The listing builds one solid part. Answer for the finished solid, in the listing's coordinates (mm). A direction names the side the tool comes from. Round coordinates to 2 decimals unless told otherwise and drop trailing zeros. Use a Markdown table: item, result. Add a question column.
Q1. Which of the six approach directions +Z, -Z, +X, -X, +Y, -Y give full straight-line access (tool end or side, diameter ignored) to faces 1 (the flat face through (104, 147, 2)), 2 (the flat face through (18.583, 98, 2)), 3 (the flat face through (231, 5, 2)), 4 (the flat face through (104, 2, 2))?
Q2. Section A-A on x = 191.5 is taken. Give the number of separate pieces and of enclosed holes in the cut face, then the cut area to 3 significant figures.
Q3. For a pull along Y with two mould halves and no side action, classify faces 5 (the flat face through (258, 60, 2)), 6 (the flat face through (18.583, 78, 2)), 7 (the flat face through (2, 30, 2)), 8 (the flat face through (0, 105, 2)) as released by +Y, released by -Y, zero draft, split by the parting line, or undercut.
Q4. Consider line 1 (X direction, y = 126.5, z = 0.85); line 2 (X direction, y = 108, z = 0.55); line 3 (Y direction, x = 16, z = 4.3). Determine where each line is inside the solid, lowest interval first.
Q5. Given pin 1 Ø1.5 at (x, z) = (3, 3) entering from +Y; pin 2 Ø2.5 at (x, z) = (234.5, 1.5) entering from +Y; pin 3 Ø2.5 at (y, z) = (3, 3.5) entering from +X, each flat-ended and moving along its own axis, determine where each tip first touches the part or whether it passes through.
from build123d import *

# Parameters (mm, degrees)
CROQUIS1_W              = 219.410669775
CROQUIS1_H              = 5
SALIENTE_EXTRUIR1_DEPTH = 5


with BuildPart() as part:
    # Croquis1 → Saliente-Extruir1 (new body)
    with BuildSketch(Plane.XY):
        Polygon((52, 0), (104, 0), (104, 5), (156, 5), (156, 0), (208, 0), (208, 5), (255, 5), (255, 30), (260, 30), (260, 60), (255, 60), (255, 90), (260, 90), (260, 120), (255, 120), (255, 145), (208, 145), (208, 150), (156, 150), (156, 145), (104, 145), (104, 150), (52, 150), (52, 145), (5, 145), (5, 120), (0, 120), (0, 90), (5, 90), (5, 60), (0, 60), (0, 30), (5, 30), (5, 5), (52, 5), align=None)
        with Locations((128.287883766, 128.217905572)):
            Rectangle(CROQUIS1_W, CROQUIS1_H, mode=Mode.SUBTRACT)
        with Locations((128.287883766, 118.217905572)):
            Rectangle(CROQUIS1_W, CROQUIS1_H, mode=Mode.SUBTRACT)
        with Locations((128.287883766, 108.217905572)):
            Rectangle(CROQUIS1_W, CROQUIS1_H, mode=Mode.SUBTRACT)
        with Locations((128.287883766, 98.217905572)):
            Rectangle(CROQUIS1_W, CROQUIS1_H, mode=Mode.SUBTRACT)
        with Locations((128.287883766, 88.217905572)):
            Rectangle(CROQUIS1_W, CROQUIS1_H, mode=Mode.SUBTRACT)
        with Locations((128.287883766, 78.217905572)):
            Rectangle(CROQUIS1_W, CROQUIS1_H, mode=Mode.SUBTRACT)
        with Locations((128.287883766, 68.217905572)):
            Rectangle(CROQUIS1_W, CROQUIS1_H, mode=Mode.SUBTRACT)
    extrude(amount=SALIENTE_EXTRUIR1_DEPTH)


solid = part.part
Checked values:
| question | item | result |
|---|---|---|
| 1 | face 1 | +Z, -Z, +Y |
| 1 | face 2 | +Z, -Z |
| 1 | face 3 | +Z, -Z, +X, -Y |
| 1 | face 4 | +Z, -Z, -Y |
| 2 | separate pieces | 8 |
| 2 | enclosed holes | 0 |
| 2 | area | 575 mm2 |
| 3 | face 5 | undercut |
| 3 | face 6 | undercut |
| 3 | face 7 | released by -Y |
| 3 | face 8 | zero draft |
| 4 | line 1 | x = 5 to 18.58, 237.99 to 255 |
| 4 | line 2 | x = 0 to 18.58, 237.99 to 260 |
| 4 | line 3 | y = 5 to 145 |
| 5 | pin 1 | stops at y = 120 |
| 5 | pin 2 | stops at y = 145 |
| 5 | pin 3 | stops at x = 208 |
